```python
from build123d import *

# Parameters (mm, degrees)
SKETCH1_R           = 25
BOSS_EXTRUDE1_DEPTH = 7
SKETCH2_R           = 24
CUT_EXTRUDE1_DEPTH  = 6
FILLET1_R           = 1


with BuildPart() as part:
    # Sketch1 → Boss-Extrude1 (new body)
    with BuildSketch(Plane(origin=(0, 0, 0), x_dir=(1, 0, 0), z_dir=(0, 1, 0))):
        Circle(SKETCH1_R)
    extrude(amount=BOSS_EXTRUDE1_DEPTH)

    # Sketch2 → Cut-Extrude1 (cut)
    with BuildSketch(Plane(origin=(0, 7, 0), x_dir=(1, 0, 0), z_dir=(0, 1, 0))):
        Circle(SKETCH2_R)
    extrude(amount=-CUT_EXTRUDE1_DEPTH, mode=Mode.SUBTRACT)

    # Fillet1
    fillet1_edges = [part.edges().sort_by_distance(p)[0] for p in [
        (-25, 0, 0),
        (-24, 1, 0),
    ]]
    fillet(fillet1_edges, radius=FILLET1_R)


solid = part.part
```
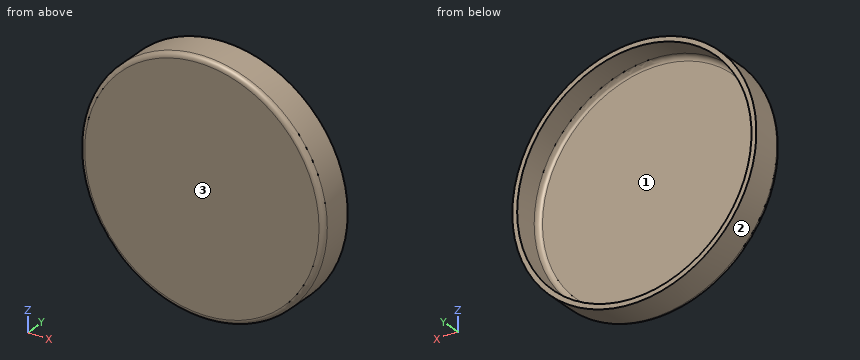
For this review, take the finished solid that the model builds, in its own axes (mm). Face numbers are marked on the shaded views. Coordinates: 2 decimals unless noted, no trailing zeros. Order: outer loops, then holes, each group sorted by start corner. A loop starts at its lowest first (then second) coordinate and runs counter-clockwise, first axis right, second up. Notation, with made-up numbers: (-17.5, -7.5) -> (26.5, -7.5) arc R16 ccw to (26.5, 14.5) -> close; hole circle Ø5 at (-40, -9.75). An arc over 180 degrees is marked (long way). Answer as CSV lines item,"result".
Q1. We need section A-A (z = 0). State the section outline as (x, y) points, plus the area to 3 significant figures.
Model answer:
outline,"(-25, 1) arc R1 ccw to (-24, 0) -> (24, 0) arc R1 ccw to (25, 1) -> (25, 7) -> (24, 7) -> (24, 2) arc R1 cw to (23, 1) -> (-23, 1) arc R1 cw to (-24, 2) -> (-24, 7) -> (-25, 7) -> close"
area,"62.0 mm2"
Q2. We need section C-C (y = 5.5). State the section outline as (x, z) points.
Model answer:
outline,"circle Ø50 at (0, 0); hole circle Ø48 at (0, 0)"
Q3. Clearance check with flat-ended pins moving along their axes: pin 1 Ø1.5 at (x, y) = (9.5, 3.5) entering from -Z; pin 2 Ø3 at (x, y) = (-2, 5) entering from +Z (3 decimals); pin 3 Ø1 at (x, y) = (-4, 3.5) entering from -Z. State where each tip first meets the part, or that it passes through.
Model answer:
pin 1,"stops at z = -23.42"
pin 2,"stops at z = 24.995"
pin 3,"stops at z = -24.75"
Q4. Draft analysis for pull direction X (two halves, no side actions). For the marked faces 1, 2 and 3, state which applies: released by +X, released by -X, zero draft, split by the parting line, or undercut.
Model answer:
face 1,"undercut"
face 2,"split by the parting line"
face 3,"zero draft"
Q5. We need section B-B (x = 0). State the section outline as (y, z) points, plus the area to 3 significant figures.
Model answer:
outline,"(0, -24) arc R1 ccw to (1, -25) -> (7, -25) -> (7, -24) -> (2, -24) arc R1 cw to (1, -23) -> (1, 23) arc R1 cw to (2, 24) -> (7, 24) -> (7, 25) -> (1, 25) arc R1 ccw to (0, 24) -> close"
area,"62.0 mm2"
Q6. Wall thickness on line 1 along X through (y, z) = (3.75, 0); line 2 along Y through (x, z) = (-3, -7): over which ranges is each line inside the solid? List them lowest first. Write a range as [from, to].
Model answer:
line 1,"x = [-25, -24], [24, 25]"
line 2,"y = [0, 1]"
